```python
from build123d import *

# Parameters (mm, degrees)
SKETCH_1_W          = 105
SKETCH_1_H          = 35
EXTRUDE_1_DEPTH     = 3
SKETCH_3_W          = 24
SKETCH_3_H          = 35
EXTRUDE_2_DEPTH     = 3
SKETCH_4_W          = 95
SKETCH_4_H          = 135
EXTRUDE_3_DEPTH     = 3
SKETCH_5_R          = 1.65
CUT_EXTRUDE_1_DEPTH = 172.052623482
SKETCH_6_R          = 1.65
CUT_EXTRUDE_2_DEPTH = 40


with BuildPart() as part:
    # 草图1 → 凸台-拉伸1 (new body)
    with BuildSketch(Plane.XY):
        with Locations((52.5, -17.5)):
            Rectangle(SKETCH_1_W, SKETCH_1_H)
    extrude(amount=EXTRUDE_1_DEPTH)

    # 草图3 → 凸台-拉伸2 (add)
    with BuildSketch(Plane.XY.offset(3)):
        with Locations((-12, -17.5)):
            Rectangle(SKETCH_3_W, SKETCH_3_H)
    extrude(amount=-EXTRUDE_2_DEPTH)

    # 草图4 → 凸台-拉伸3 (add)
    with BuildSketch(Plane.XY.offset(3)):
        with Locations((30.5, 67.5)):
            Rectangle(SKETCH_4_W, SKETCH_4_H)
    extrude(amount=-EXTRUDE_3_DEPTH)

    # 草图5 → 切除-拉伸1 (cut, through all)
    with BuildSketch(Plane(origin=(0, 0, 0), x_dir=(-1, 0, 0), z_dir=(0, 0, -1))):
        with Locations((-87, -7)):
            Circle(SKETCH_5_R)
        with Locations((-96, -16)):
            Circle(SKETCH_5_R)
        with Locations((-87, -25)):
            Circle(SKETCH_5_R)
        with Locations((-78, -16)):
            Circle(SKETCH_5_R)
    extrude(amount=-CUT_EXTRUDE_1_DEPTH, mode=Mode.SUBTRACT)

    # 草图6 → 切除-拉伸2 (cut)
    with BuildSketch(Plane.XY.offset(3)):
        with Locations((35, 1)):
            Circle(SKETCH_6_R)
        with Locations((35, 11)):
            Circle(SKETCH_6_R)
        with Locations((71, 1)):
            Circle(SKETCH_6_R)
        with Locations((71, 11)):
            Circle(SKETCH_6_R)
        with Locations((47, -17)):
            Circle(SKETCH_6_R)
        with Locations((59, -17)):
            Circle(SKETCH_6_R)
        with Locations((59, -3)):
            Circle(SKETCH_6_R)
        with Locations((47, -3)):
            Circle(SKETCH_6_R)
        with Locations((59, 11)):
            Circle(SKETCH_6_R)
        with Locations((47, 11)):
            Circle(SKETCH_6_R)
    extrude(amount=-CUT_EXTRUDE_2_DEPTH, mode=Mode.SUBTRACT)


solid = part.part
```
The listing builds one solid part. Answer for the finished solid, in the listing's coordinates (mm). Coordinates: 2 decimals unless noted, no trailing zeros. Write each loop counter-clockwise with the first axis right and the second up, starting at its lowest first coordinate (ties: lowest second). Pieces come first, ordered by that corner, then holes. Notation, with made-up numbers: (-36, 7) - (6, 7) arc R21 cw to (6, 40) - close; hole circle Ø9 at (12, 71). An arc over 180 degrees is marked (long way). Return JSON: item names as keys, results as strings. Group by question number.
1. Given pin 1 (0.9 mm diameter, centred on x = 97, z = 1.5, fed in from +Y); pin 2 (0.9 mm diameter, centred on y = 46.5, z = 1, fed in from -X), each flat-ended and moving along its own axis, determine where each tip first touches the part or whether it passes through.
2. Determine the mould class of faces 1 (the cylindrical face through (69.784, 2.115, 1.521)), 2 (the flat face through (40, 51, 3)) for opening direction X: released by +X, released by -X, zero draft, split by the parting line, or undercut.
3. A cutting plane is placed at A-A, the plane z = 2.1. Give the number of separate pieces and of enclosed holes in the cut face, plus the area to 3 significant figures.
4. A cutting plane is placed at B-B, the plane x = 82. Determine the outline of the cut face in (y, z), plus the area to 3 significant figures.
5. Straight lines are drawn through the part: L1, parallel to Y at x = 35, z = 1.8; L2, parallel to Y at x = 59, z = 1.3; L3, parallel to X at y = 19.5, z = 1.15. For each, find the intervals that lie inside material, in ascending order.
6. A cutting plane is placed at C-C, the plane y = 16. Determine the outline of the cut face in (x, z), plus the area to 3 significant figures.
Ans:
{
 "1": {"pin 1": "y = 0", "pin 2": "x = -17"},
 "2": {"face 1": "undercut", "face 2": "zero draft"},
 "3": {"separate pieces": "1", "enclosed holes": "14", "area": "17,200 mm²"},
 "4": {"outline": "(-35, 0) - (0, 0) - (0, 3) - (-35, 3) - close", "area": "105 mm²"},
 "5": {"L1": "-35 to -0.65, 2.65 to 9.35, 12.65 to 135", "L2": "-35 to -18.65, -15.35 to -4.65, -1.35 to 9.35, 12.65 to 135", "L3": "-17 to 78"},
 "6": {"outline": "(-17, 0) - (78, 0) - (78, 3) - (-17, 3) - close", "area": "285 mm²"}
}
